Design review of the part shown in the three views and the two pictorial views. Dimensions are in mm from the part's minimum x, y and z. A direction names the side the tool comes from. Round coordinates to 2 decimals unless told otherwise and drop trailing zeros. Order: outer loops, then holes, each group sorted by start corner. A loop starts at its lowest first (then second) coordinate and runs counter-clockwise, first axis right, second up. Notation, with made-up numbers: M -30.5,4.25 L 13.5,4.25 A17 ccw 13.5,22.25 Z; hole C -28.75,-28 d10. An arc over 180 degrees is marked long. Use a Markdown table: item, result. Add a question column.
(1) For pin 1 (20 mm diameter, centred on x = 24, z = 19.5, fed in from -Y); pin 2 (2 mm diameter, centred on x = 24, y = 6.5, fed in from -Z); pin 3 (2 mm diameter, centred on x = 34, z = 7, fed in from -Y), all flat-tipped, find the tip position at first contact; note any pin that passes through.
(2) Machinability: for the marked faces 1 and 2, which of the approach directions +Z, -Z, +X, -X, +Y, -Y give a long, thin tool a straight path to every point of the face, cutting with its end or side? Answer none if there is none.
(3) The part is to be moulded in two halves that separate along Z. For the marked faces 3, 4 and 5, say which applies: released by +Z, released by -Z, zero draft, split by the parting line, or undercut.
(4) Take a section at A-A (y = 9.25). Write out the cut boundary in (x, z) (1 decimal).
(5) Take a section at C-C (y = 16.5). Write out the cut boundary in (x, z).
(6) To check wall thickness, follow probe 1 along Y at (x, z) = (32, 25); probe 2 along X at (y, z) = (11.25, 32.5) (1 decimal); probe 3 along Z at (x, y) = (10, 11.5) (1 decimal). State the ranges of each line that lie inside material, in increasing order. Write a range as from..to.
(7) Take a section at B-B (y = 13.5). Write out the cut boundary in (x, z) (1 decimal).
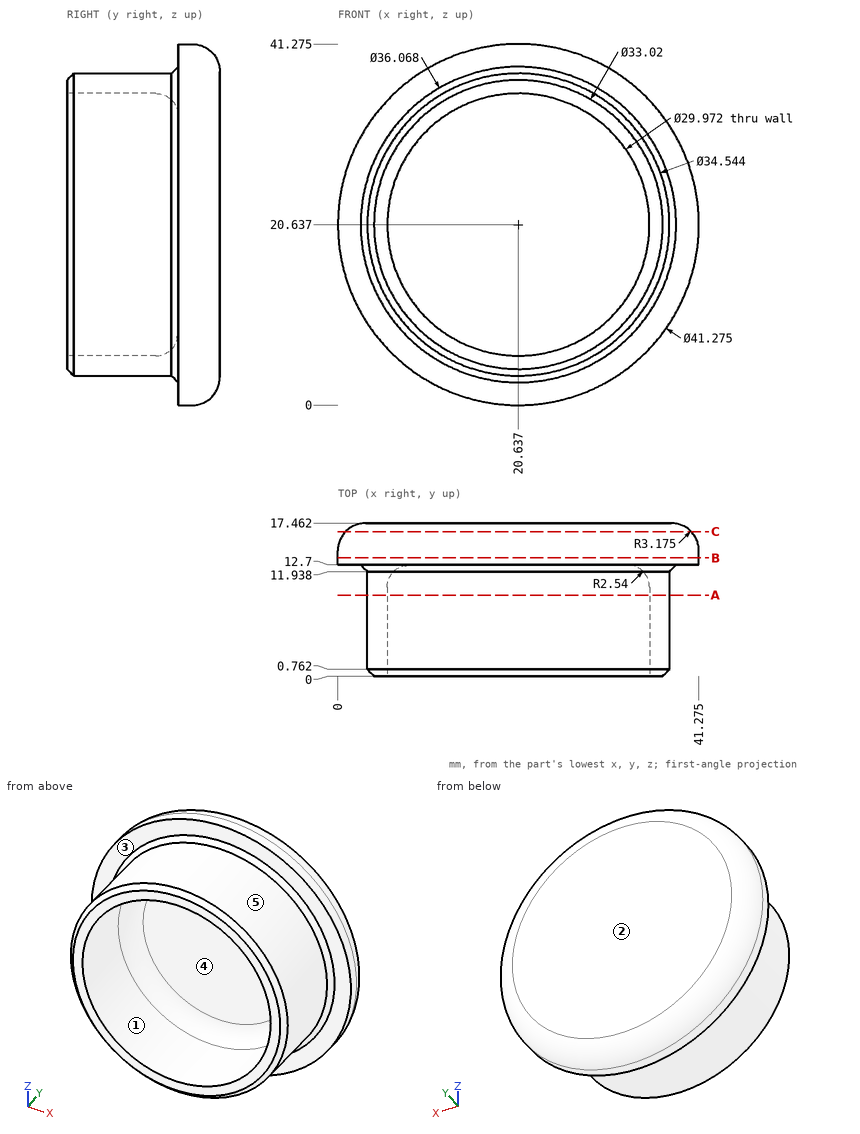
Verdict:
| question | item | result |
|---|---|---|
| 1 | pin 1 | stops at y = 12.45 |
| 1 | pin 2 | stops at z = 3.53 |
| 1 | pin 3 | stops at y = 12.7 |
| 2 | face 1 | -Y |
| 2 | face 2 | +Z, -Z, +X, -X, +Y |
| 3 | face 3 | zero draft |
| 3 | face 4 | undercut |
| 3 | face 5 | split by the parting line |
| 4 | outline | C 20.6,20.6 d34.5; hole C 20.6,20.6 d30 |
| 5 | outline | C 20.64,20.64 d39.48 |
| 6 | probe 1 | y = 12.7..17.46 |
| 6 | probe 2 | x = 8.1..11.9, 29.4..33.2 |
| 6 | probe 3 | z = 7..10.6, 30.6..34.2 |
| 7 | outline | C 20.6,20.6 d41.3 |
